Can you work these out from the model? Positions are in its coordinate system, mm. A direction names the side the tool comes from. Give positions to 0.01 mm unless a question says otherwise; leave off trailing zeros. Write each loop counter-clockwise with the first axis right and the second up, starting at its lowest first coordinate (ties: lowest second). Pieces come first, ordered by that corner, then holes. Notation, with made-up numbers: (39, 71.5) -> (69, 71.5) arc R18 cw to (69, 92.5) -> close; hole circle Ø1 at (17.5, 78.5). An arc over 180 degrees is marked (long way). One line per item, written item: value.
from build123d import *

# Parameters (mm, degrees)
SKETCH1_W           = 25
SKETCH1_H           = 25
SKETCH1_W_2         = 21.8
SKETCH1_H_2         = 21.8
BOSS_EXTRUDE1_DEPTH = 300
SKETCH2_W           = 40
SKETCH2_H           = 40
BOSS_EXTRUDE2_DEPTH = 3
CUT_EXTRUDE1_REACH  = 303.703
SKETCH3_R           = 3
CUT_EXTRUDE2_REACH  = 303.921
SKETCH4_R           = 2


with BuildPart() as part:
    # Sketch1 → Boss-Extrude1 (new body)
    with BuildSketch(Plane(origin=(0, 0, 0), x_dir=(1, 0, 0), z_dir=(0, 1, 0))):
        Rectangle(SKETCH1_W, SKETCH1_H)
        Rectangle(SKETCH1_W_2, SKETCH1_H_2, mode=Mode.SUBTRACT)
    extrude(amount=BOSS_EXTRUDE1_DEPTH)

    # Sketch2 → Boss-Extrude2 (add)
    with BuildSketch(Plane.XZ):
        with Locations((0, 7.5)):
            Rectangle(SKETCH2_W, SKETCH2_H)
    extrude(amount=BOSS_EXTRUDE2_DEPTH)

    # Sketch3 → Cut-Extrude1 (cut, up to next)
    with BuildSketch(Plane.XY.offset(12.5), mode=Mode.PRIVATE) as cut_extrude1_sk1:
        with Locations((0, 187)):
            Circle(SKETCH3_R)
    cut_extrude1_tool1 = extrude(cut_extrude1_sk1.sketch, amount=-CUT_EXTRUDE1_REACH, mode=Mode.PRIVATE) & part.part
    # Sketch3 → Cut-Extrude1 (cut, up to next)
    with BuildSketch(Plane.XY.offset(12.5), mode=Mode.PRIVATE) as cut_extrude1_sk2:
        with Locations((0, 282)):
            Circle(SKETCH3_R)
    cut_extrude1_tool2 = extrude(cut_extrude1_sk2.sketch, amount=-CUT_EXTRUDE1_REACH, mode=Mode.PRIVATE) & part.part
    add(cut_extrude1_tool1.solids().sort_by_distance((0, 187, 12.5))[0], mode=Mode.SUBTRACT)
    add(cut_extrude1_tool2.solids().sort_by_distance((0, 282, 12.5))[0], mode=Mode.SUBTRACT)

    # Sketch4 → Cut-Extrude2 (cut, up to next)
    with BuildSketch(Plane(origin=(0, 0, 0), x_dir=(1, 0, 0), z_dir=(0, 1, 0)), mode=Mode.PRIVATE) as cut_extrude2_sk1:
        with Locations(Location((0, -20.5, 0), (0, 0, 270))):
            Circle(SKETCH4_R)
    cut_extrude2_tool1 = extrude(cut_extrude2_sk1.sketch, amount=-CUT_EXTRUDE2_REACH, mode=Mode.PRIVATE) & part.part
    add(cut_extrude2_tool1.solids().sort_by_distance((0, 0, 20.5))[0], mode=Mode.SUBTRACT)


solid = part.part
1) If we section it at C-C (x = 7): Write out the boundary of the cut face in (y, z).
Answer list:
outline: (-3, -12.5) -> (300, -12.5) -> (300, -10.9) -> (0, -10.9) -> (0, 10.9) -> (300, 10.9) -> (300, 12.5) -> (0, 12.5) -> (0, 27.5) -> (-3, 27.5) -> close
2) We'd pull the mould along Z, two halves only. Please class faces 1 (the face through (0, 148, 12.5)), 2 (the face through (0, 148, -10.9)), 3 (the face through (0, 148, 10.9)), 4 (the face through (0, 285, 12)): released by +Z, released by -Z, zero draft, split by the parting line, or undercut.
Answer list:
face 1: released by +Z
face 2: undercut
face 3: undercut
face 4: zero draft
3) If we section it at B-B (y = 247.5): Write out the boundary of the cut face in (x, z).
Answer list:
outline: (-12.5, -12.5) -> (12.5, -12.5) -> (12.5, 12.5) -> (-12.5, 12.5) -> close; hole (-10.9, -10.9) -> (10.9, -10.9) -> (10.9, 10.9) -> (-10.9, 10.9) -> close
4) If we section it at D-D (z = 15): Write out the boundary of the cut face in (x, y), and give its area (3 significant figures).
Answer list:
outline: (-20, -3) -> (20, -3) -> (20, 0) -> (-20, 0) -> close
area: 120 mm^2
5) Will these pins go through, and if not, where does the flat tip stop? pin 1 (24 mm diameter, centred on x = 3.5, z = 0.5, fed in from +Y); pin 2 (6.5 mm diameter, centred on y = 189, z = 4, fed in from -X); pin 3 (5.5 mm diameter, centred on x = 0, y = 282, fed in from +Z); pin 4 (5 mm diameter, centred on y = 128.5, z = 1.5, fed in from +X).
Answer list:
pin 1: stops at y = 300
pin 2: stops at x = -12.5
pin 3: stops at z = -10.9
pin 4: stops at x = 12.5
6) For faces 5 (the face through (-12.5, 148, 0)), 6 (the face through (12.5, 148, 0)), 7 (the face through (10.9, 148, 0)), which set-ups out of +Z, -Z, +X, -X, +Y, -Y let a thin tool reach every point of the face, with its end or its side?
Answer list:
face 5: +Z, -Z, -X, +Y
face 6: +Z, -Z, +X, +Y
face 7: +Y
7) I need wall thicknesses on L1, parallel to Y at x = 0, z = 12; L2, parallel to X at y = 178.5, z = 9.5; L3, parallel to X at y = 282, z = 11.8. Which ranges of each line are inside material? Lowest first, please.
Answer list:
L1: y = -3 to 184, 190 to 279, 285 to 300
L2: x = -12.5 to -10.9, 10.9 to 12.5
L3: x = -12.5 to -3, 3 to 12.5
8) If we section it at A-A (y = 187): Write out the boundary of the cut face in (x, z).
Answer list:
outline: (-12.5, -12.5) -> (12.5, -12.5) -> (12.5, 12.5) -> (3, 12.5) -> (3, 10.9) -> (10.9, 10.9) -> (10.9, -10.9) -> (-10.9, -10.9) -> (-10.9, 10.9) -> (-3, 10.9) -> (-3, 12.5) -> (-12.5, 12.5) -> close
